Work out the finished part from the listing and answer in its coordinate system (mm). Round coordinates to 2 decimals unless told otherwise and drop trailing zeros. Write each loop counter-clockwise with the first axis right and the second up, starting at its lowest first coordinate (ties: lowest second). Pieces come first, ordered by that corner, then holes. Notation, with made-up numbers: (22, 26.5) - (58, 26.5) arc R3 ccw to (58, 31.5) - close; hole circle Ø2 at (64, 87). An arc over 180 degrees is marked (long way). Answer as a JSON object with one key per item and string values.
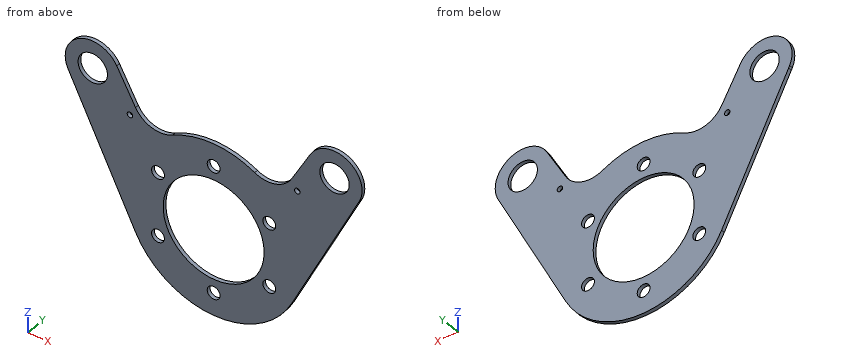
```python
from build123d import *

# Parameters (mm, degrees)
F2_R     = 3.5
F2_R_2   = 27.5
F2_R_3   = 1.5
F2_R_4   = 8
F3_DEPTH = 2


with BuildPart() as f3:
    # F2 (on Front) → F3 (new body)
    with BuildSketch(Plane.XZ):
        with BuildLine():
            Line((-42.53072, 47.831513), (-52.759336, 66.173364))
            ThreePointArc((-52.759336, 66.173364), (-72.578902, 72.278632), (-79.555119, 52.748606))
            Line((-79.555119, 52.748606), (-78.960552, 51.561851))
            Line((-78.960552, 51.561851), (-42.468246, -21.276702))
            ThreePointArc((-42.468246, -21.276702), (0, -47.5), (42.468246, -21.276702))
            Line((42.468246, -21.276702), (78.960552, 51.561851))
            Line((78.960552, 51.561851), (79.555119, 52.748606))
            ThreePointArc((79.555119, 52.748606), (72.578902, 72.278632), (52.759336, 66.173364))
            Line((52.759336, 66.173364), (42.53072, 47.831513))
            ThreePointArc((42.53072, 47.831513), (33.660405, 40.74614), (22.366885, 41.904325))
            ThreePointArc((22.366885, 41.904325), (0, 47.5), (-22.366885, 41.904325))
            ThreePointArc((-22.366885, 41.904325), (-33.660405, 40.74614), (-42.53072, 47.831513))
        make_face()
        with Locations((-30.310889, -17.5)):
            Circle(F2_R, mode=Mode.SUBTRACT)
        with Locations((0, -35)):
            Circle(F2_R, mode=Mode.SUBTRACT)
        with Locations((30.310889, -17.5)):
            Circle(F2_R, mode=Mode.SUBTRACT)
        Circle(F2_R_2, mode=Mode.SUBTRACT)
        with Locations((-45.577269, 42.382158)):
            Circle(F2_R_3, mode=Mode.SUBTRACT)
        with Locations((-30.310889, 17.5)):
            Circle(F2_R, mode=Mode.SUBTRACT)
        with Locations((-65.859944, 58.867607)):
            Circle(F2_R_4, mode=Mode.SUBTRACT)
        with Locations((30.310889, 17.5)):
            Circle(F2_R, mode=Mode.SUBTRACT)
        with Locations((0, 35)):
            Circle(F2_R, mode=Mode.SUBTRACT)
        with Locations((45.577269, 42.382158)):
            Circle(F2_R_3, mode=Mode.SUBTRACT)
        with Locations((65.859944, 58.867607)):
            Circle(F2_R_4, mode=Mode.SUBTRACT)
    extrude(amount=-F3_DEPTH)


solid = f3.part
```
Item 1: A cutting plane is placed at A-A (x = 0). Write down the section's boundary in (y, z), and give its area (3 significant figures).
Results found:
{"outline": "(0, -47.5) - (2, -47.5) - (2, -38.5) - (0, -38.5) - close; (0, -31.5) - (2, -31.5) - (2, -27.5) - (0, -27.5) - close; (0, 27.5) - (2, 27.5) - (2, 31.5) - (0, 31.5) - close; (0, 38.5) - (2, 38.5) - (2, 47.5) - (0, 47.5) - close", "area": "52.0 mm²"}
Item 2: Consider line 1 along Z through (x, y) = (-0.5, 1.25); line 2 along X through (y, z) = (0.3, 54); line 3 along X through (y, z) = (0.2, 19.5). Determine where each line is inside the solid, lowest interval first.
Results found:
{"line 1": "-47.5 to -38.46, -31.54 to -27.5, 27.5 to 31.54, 38.46 to 47.5", "line 2": "-80.05 to -72.21, -59.51 to -45.97, 45.97 to 59.51, 72.21 to 80.05", "line 3": "-62.9 to -33.18, -27.44 to -19.39, 19.39 to 27.44, 33.18 to 62.9"}
Item 3: Each of these flat-tipped pins is pushed along its axis until it touches: P1, Ø1, axis at x = -52, y = 0.5, coming from the +Z side; P2, Ø1, axis at x = 10, y = 1.5, coming from the -Z side; P3, Ø1, axis at x = 17.5, y = 0.5, coming from the +Z side. Where does it stop, or does it pass through?
Results found:
{"P1": "z = 65.71", "P2": "z = -46.54", "P3": "z = 44.35"}
Item 4: A cutting plane is placed at C-C (x = -67.5). Write down the section's boundary in (y, z).
Results found:
{"outline": "(0, 28.69) - (2, 28.69) - (2, 51.04) - (0, 51.04) - close; (0, 66.7) - (2, 66.7) - (2, 73.78) - (0, 73.78) - close"}
Item 5: A cutting plane is placed at D-D (y = 0.45). Give the number of separate pieces and of enclosed holes in the cut face, and give its area (3 significant figures).
Results found:
{"separate pieces": "1", "enclosed holes": "11", "area": "7,960 mm²"}
Item 6: A cutting plane is placed at B-B (z = 17.5). Write down the section's boundary in (x, y), and give its area (3 significant figures).
Results found:
{"outline": "(-61.9, 0) - (-33.81, 0) - (-33.81, 2) - (-61.9, 2) - close; (-26.81, 0) - (-21.21, 0) - (-21.21, 2) - (-26.81, 2) - close; (21.21, 0) - (26.81, 0) - (26.81, 2) - (21.21, 2) - close; (33.81, 0) - (61.9, 0) - (61.9, 2) - (33.81, 2) - close", "area": "135 mm²"}
